Work out the finished part from the listing and answer in its coordinate system (mm). A direction names the side the tool comes from. Round coordinates to 2 decimals unless told otherwise and drop trailing zeros. Write each loop counter-clockwise with the first axis right and the second up, starting at its lowest first coordinate (ties: lowest second). Pieces come first, ordered by that corner, then holes. Notation, with made-up numbers: (-7.75, 45) - (23.25, 45) arc R18 ccw to (23.25, 63) - close; hole circle Ø1 at (52.25, 23). An arc over 180 degrees is marked (long way). Answer as a JSON object with one key per item and string values.
```python
from build123d import *

# Parameters (mm, degrees)
BOSS_EXTRUDE1_DEPTH = 9
SKETCH2_R           = 7.5
BOSS_EXTRUDE2_DEPTH = 21
BOSS_EXTRUDE3_DEPTH = 3.5
SKETCH4_R           = 7.5
CUT_EXTRUDE1_DEPTH  = 85.242328054


with BuildPart() as part:
    # Sketch1 → Boss-Extrude1 (new body)
    with BuildSketch(Plane(origin=(0, 0, 0), x_dir=(1, 0, 0), z_dir=(0, 1, 0))):
        with BuildLine():
            Line((-5.007194245, 0), (6.992805755, 0))
            Line((6.992805755, 0), (15.992805755, 4.683453237))
            Line((15.992805755, 4.683453237), (15.992805755, 65))
            ThreePointArc((15.992805755, 65), (0.992805755, 80), (-14.007194245, 65))
            Line((-14.007194245, 65), (-14.007194245, 4.683453237))
            Line((-14.007194245, 4.683453237), (-5.007194245, 0))
        make_face()
    extrude(amount=BOSS_EXTRUDE1_DEPTH)

    # Sketch2 → Boss-Extrude2 (add)
    with BuildSketch(Plane(origin=(0, 9, 0), x_dir=(1, 0, 0), z_dir=(0, 1, 0))):
        with BuildLine():
            ThreePointArc((15.992805755, 65), (0.992805755, 80), (-14.007194245, 65))
            Line((-14.007194245, 65), (-14.007194245, 47))
            Line((-14.007194245, 47), (15.992805755, 47))
            Line((15.992805755, 47), (15.992805755, 65))
        make_face()
        with Locations(Location((0.992805755, 65, 0), (0, 0, 90))):
            Circle(SKETCH2_R, mode=Mode.SUBTRACT)
    extrude(amount=BOSS_EXTRUDE2_DEPTH)

    # Sketch3 → Boss-Extrude3 (add, symmetric)
    with BuildSketch(Plane(origin=(0.992805755, 0, 0), x_dir=(0, 0, -1), z_dir=(1, 0, 0))):
        Polygon((0, 9), (47, 30), (47, 9), align=None)
    extrude(amount=BOSS_EXTRUDE3_DEPTH, both=True)

    # Sketch4 → Cut-Extrude1 (cut, through all)
    with BuildSketch(Plane(origin=(0, 9, 0), x_dir=(1, 0, 0), z_dir=(0, 1, 0))):
        with Locations(Location((0.992805755, 65, 0), (0, 0, 90))):
            Circle(SKETCH4_R)
    extrude(amount=-CUT_EXTRUDE1_DEPTH, mode=Mode.SUBTRACT)


solid = part.part
```
Item 1: For faces 1 (the flat face through (-8, 9, -24)), 2 (the flat face through (-9.57, 4.437, -2.375)), 3 (the flat face through (4.493, 15, -34)), determine the directions among +Z, -Z, +X, -X, +Y, -Y from which every point of the face is accessible in a straight line to the end or side of a thin tool.
Results found:
{"face 1": "+Z, -X, +Y", "face 2": "+Z, -X, +Y, -Y", "face 3": "+Z, +X, +Y"}
Item 2: A cutting plane is placed at A-A (x = 5.25). Write down the section's boundary in (y, z), and give its area (3 significant figures).
Results found:
{"outline": "(0, -79.38) - (30, -79.38) - (30, -71.17) - (0, -71.17) - close; (0, -58.83) - (30, -58.83) - (30, -47) - (9, -47) - (9, 0) - (0, 0) - close", "area": "1,020 mm²"}
Item 3: A cutting plane is placed at D-D (x = -10). Write down the section's boundary in (y, z).
Results found:
{"outline": "(0, -75.21) - (30, -75.21) - (30, -47) - (9, -47) - (9, -2.6) - (0, -2.6) - close"}
Item 4: Consider line 1 along X through (y, z) = (5.75, -65); line 2 along Y through (x, z) = (-5, -36); line 3 along Z through (x, y) = (3.5, 3.5). Determine where each line is inside the solid, lowest interval first.
Results found:
{"line 1": "-14.01 to -6.51, 8.49 to 15.99", "line 2": "0 to 9", "line 3": "-79.79 to -72.07, -57.93 to 0"}
Item 5: A cutting plane is placed at C-C (z = -8). Write down the section's boundary in (x, y).
Results found:
{"outline": "(-14.01, 0) - (15.99, 0) - (15.99, 9) - (4.49, 9) - (4.49, 12.57) - (-2.51, 12.57) - (-2.51, 9) - (-14.01, 9) - close"}
Item 6: Each of these flat-tipped pins is pushed along its axis until it touches: P1, Ø5, axis at x = 10.5, y = 13.5, coming from the +Z side; P2, Ø12, axis at x = -10.5, z = -19, coming from the +Y side; P3, Ø8, axis at x = 4, y = 14, coming from the +Z side. Where does it stop, or does it pass through?
Results found:
{"P1": "z = -47", "P2": "y = 9", "P3": "z = -2.24"}
Item 7: A cutting plane is placed at B-B (y = 6). Write down the section's boundary in (x, z).
Results found:
{"outline": "(-14.01, -65) arc R15 ccw to (15.99, -65) - (15.99, -4.68) - (6.99, 0) - (-5.01, 0) - (-14.01, -4.68) - close; hole circle Ø15 at (0.99, -65)"}
